For this review, take the finished solid that the model builds, in its own axes (mm). A direction names the side the tool comes from. Coordinates: 2 decimals unless noted, no trailing zeros. Loops run counter-clockwise (first coordinate to the right, second up) from the corner with the lowest first, then second, coordinate; pieces in that order, holes last. Notation, with made-up numbers: (-9, -28.75) - (15, -28.75) arc R19 ccw to (15, 7.25) - close; hole circle Ø1 at (-12.75, -17). An arc over 180 degrees is marked (long way). One line per item, written item: value. Start each with the question number.
1. The part is to be moulded in two halves that separate along Y. For faces 5 (the face through (15.5, 0, 18)), 6 (the face through (-6.4, 0.08, 28.48)), 7 (the face through (0, -5.5, 11)), say which applies: released by +Y, released by -Y, zero draft, split by the parting line, or undercut.
2. For faces 1 (the face through (11, 0, 9)), 2 (the face through (11, 0, 21)), 3 (the face through (-13, 0, 17)), 4 (the face through (-10.2, -0.4, 23)), list the 3-axis set-ups (+Z, -Z, +X, -X, +Y, -Y) from which the entire face can be reached by the end or side of a thin tool; tool diameter is ignored.
3. To check wall thickness, follow line 1 (Z direction, x = 5, y = -1.25); line 2 (Z direction, x = -6, y = 3.75); line 3 (X direction, y = -3.75, z = 12). State the ranges of each line that lie inside material, in increasing order. Write a range as from..to.
4. Take a section at C-C, the plane x = -8. State the section outline as (y, z) points.
5. Take a section at B-B, the plane z = 11.25. State the section outline as (x, y) points.
6. Take a section at A-A, the plane x = -3. State the section outline as (y, z) points, and give its area (3 significant figures).
7. Insertion check: pin 1 (3.5 mm diameter, centred on x = -12, y = -2, fed in from +Z); pin 2 (10 mm diameter, centred on x = 12, z = 20, fed in from +Y); pin 3 (2 mm diameter, centred on x = -7.5, y = -2.5, fed in from +Z); pin 4 (5.5 mm diameter, centred on y = 2, z = 12.5, fed in from +X). Each pin has a flat end and moves straight along its axis. Give the tip position at first contact, or say it passes through.
```python
from build123d import *

# Parameters (mm, degrees)
SKETCH2_W           = 31
SKETCH2_H           = 11
SKETCH2_R           = 1.9
BOSS_EXTRUDE1_DEPTH = 23
SKETCH2_2_R         = 1.9
BOSS_EXTRUDE2_DEPTH = 30
SKETCH3_W           = 4.5
SKETCH3_H           = 11
CUT_EXTRUDE1_DEPTH  = 4
CUT_EXTRUDE2_START  = -6
SKETCH3_5_W         = 4.5
SKETCH3_5_H         = 11
CUT_EXTRUDE2_DEPTH  = 23.275431031
BOSS_EXTRUDE3_DEPTH = 4


with BuildPart() as part:
    # Sketch2 → Boss-Extrude1 (new body)
    with BuildSketch(Plane.XY):
        Rectangle(SKETCH2_W, SKETCH2_H)
        with Locations((-4.5, 0)):
            Circle(SKETCH2_R, mode=Mode.SUBTRACT)
    extrude(amount=BOSS_EXTRUDE1_DEPTH)

    # Sketch2_2 → Boss-Extrude2 (add)
    with BuildSketch(Plane.XY):
        with Locations((-4.5, 0)):
            Circle(SKETCH2_2_R)
    extrude(amount=BOSS_EXTRUDE2_DEPTH)

    # Sketch3 → Cut-Extrude1 (cut)
    with BuildSketch(Plane.XY.offset(23)):
        with Locations((-13.25, 0)):
            Rectangle(SKETCH3_W, SKETCH3_H)
        with Locations((13.25, 0)):
            Rectangle(SKETCH3_W, SKETCH3_H)
    extrude(amount=-CUT_EXTRUDE1_DEPTH, mode=Mode.SUBTRACT)

    # Sketch3_5 → Cut-Extrude2 (cut, through all)
    with BuildSketch(Plane.XY.offset(23).offset(CUT_EXTRUDE2_START)):
        with Locations((-13.25, 0)):
            Rectangle(SKETCH3_5_W, SKETCH3_5_H)
        with Locations((13.25, 0)):
            Rectangle(SKETCH3_5_W, SKETCH3_5_H)
    extrude(amount=-CUT_EXTRUDE2_DEPTH, mode=Mode.SUBTRACT)

    # Sketch4 → Boss-Extrude3 (add)
    with BuildSketch(Plane.XY.offset(23)):
        with BuildLine():
            ThreePointArc((-6.4, 0), (-4.5, 1.9), (-2.6, 0))
            Line((-2.6, 0), (1, 0))
            ThreePointArc((1, 0), (0.856071321, 1.25), (0.431818182, 2.434577873))
            ThreePointArc((0.431818182, 2.434577873), (-5.75, 5.356071321), (-10, 0))
            Line((-10, 0), (-6.4, 0))
        make_face()
        with BuildLine():
            Line((1, 0), (-2.6, 0))
            ThreePointArc((-2.6, 0), (-4.5, -1.9), (-6.4, 0))
            Line((-6.4, 0), (-10, 0))
            ThreePointArc((-10, 0), (-5.75, -5.356071321), (0.431818182, -2.434577873))
            ThreePointArc((0.431818182, -2.434577873), (0.856071321, -1.25), (1, 0))
        make_face()
        with BuildLine():
            ThreePointArc((-6.4, 0), (-4.5, -1.9), (-2.6, 0))
            Line((-2.6, 0), (-6.4, 0))
        make_face()
        with BuildLine():
            Line((-6.4, 0), (-2.6, 0))
            ThreePointArc((-2.6, 0), (-4.5, 1.9), (-6.4, 0))
        make_face()
        with BuildLine():
            ThreePointArc((0.431818182, 2.434577873), (0.856071321, 1.25), (1, 0))
            Line((1, 0), (3.5, 0))
            ThreePointArc((3.5, 0), (2.553953901, 1.95837363), (0.431818182, 2.434577873))
        make_face()
        with BuildLine():
            Line((3.5, 0), (1, 0))
            ThreePointArc((1, 0), (0.856071321, -1.25), (0.431818182, -2.434577873))
            ThreePointArc((0.431818182, -2.434577873), (2.553953901, -1.95837363), (3.5, 0))
        make_face()
    extrude(amount=BOSS_EXTRUDE3_DEPTH)


solid = part.part
```
Solutions:
1. face 5: zero draft
1. face 6: split by the parting line
1. face 7: released by -Y
2. face 1: -Z, +X, +Y, -Y
2. face 2: +Z, +X, +Y, -Y
2. face 3: -Z, -X, +Y, -Y
2. face 4: +Z, -X
3. line 1: 0..23
3. line 2: 0..27
3. line 3: -11..11
4. outline: (-5.5, 0) - (5.5, 0) - (5.5, 23) - (4.24, 23) - (4.24, 27) - (-4.24, 27) - (-4.24, 23) - (-5.5, 23) - close
5. outline: (-11, -5.5) - (11, -5.5) - (11, 5.5) - (-11, 5.5) - close
6. outline: (-5.5, 0) - (5.5, 0) - (5.5, 23) - (5.29, 23) - (5.29, 27) - (1.17, 27) - (1.17, 30) - (-1.17, 30) - (-1.17, 27) - (-5.29, 27) - (-5.29, 23) - (-5.5, 23) - close
6. area: 302 mm2
7. pin 1: z = 23
7. pin 2: y = 5.5
7. pin 3: z = 27
7. pin 4: x = 11
